from build123d import *

# Parameters (mm, degrees)
SKETCH1_R           = 2.5
SKETCH1_R_2         = 1.5
BOSS_EXTRUDE1_DEPTH = 310
SKETCH2_R           = 1.503835311
BOSS_EXTRUDE2_DEPTH = 5
LPATTERN1_COUNT     = 3
LPATTERN1_PITCH     = 30
SKETCH3_R           = 1.791065429
BOSS_EXTRUDE3_DEPTH = 5


with BuildPart() as part:
    # Sketch1 → Boss-Extrude1 (new body)
    with BuildSketch(Plane(origin=(0, 0, 0), x_dir=(1, 0, 0), z_dir=(0, 1, 0))):
        Circle(SKETCH1_R)
        Circle(SKETCH1_R_2, mode=Mode.SUBTRACT)
    extrude(amount=BOSS_EXTRUDE1_DEPTH)

    # Sketch2 → Boss-Extrude2 (add)
    with BuildSketch(Plane.XY):
        with Locations((0, 84.914129816)):
            Circle(SKETCH2_R)
    boss_extrude2 = extrude(amount=BOSS_EXTRUDE2_DEPTH)

    # LPattern1: Boss-Extrude2 ×3
    with Locations(*[(0, i * LPATTERN1_PITCH, 0) for i in range(1, LPATTERN1_COUNT)]):
        add(boss_extrude2)

    # Sketch3 → Boss-Extrude3 (add)
    with BuildSketch(Plane.XY):
        with Locations((0, 273.450822339)):
            Circle(SKETCH3_R)
    extrude(amount=BOSS_EXTRUDE3_DEPTH)


solid = part.part
CAD build for the part. Positions are in the model's coordinates, mm. A direction names the side the tool comes from. Coordinates: 2 decimals unless noted, no trailing zeros. Write each loop counter-clockwise with the first axis right and the second up, starting at its lowest first coordinate (ties: lowest second). Pieces come first, ordered by that corner, then holes. Notation, with made-up numbers: M 24,67 L 74,67 A9 cw 74,77 Z; hole C 88,7.25 d7. An arc over 180 degrees is marked long. Answer as a JSON object with one key per item and string values. Group by question number.
1) Pin check, flat tips, straight feed: pin 1 Ø2.5 at (x, z) = (0, 0) entering from -Y; pin 2 Ø3 at (x, y) = (1, 48.5) entering from +Z; pin 3 Ø1 at (x, y) = (-1, 249.5) entering from +Z. Stop position of each tip, or through.
2) Tool access for faces 1 (the face through (1.34, 152.83, -2.11)), 2 (the face through (0, 310, 2)): list every direction of +Z, -Z, +X, -X, +Y, -Y with a clear straight run to the whole face (end or side of a thin tool).
3) Wall check: line 1 (Z direction, x = 0.4, y = 29); line 2 (Z direction, x = 0, y = 179); line 3 (Y direction, x = 0.35, z = 4.75). Give the ranges that are in metal, low to high. Write a range as from..to.
4) Saw through at A-A (y = 31). Write the cut outline in (x, z).
Values follow:
{
 "1": {"pin 1": "stops at y = 83.41", "pin 2": "stops at z = 2.5", "pin 3": "stops at z = 2.45"},
 "2": {"face 1": "none", "face 2": "+Z, -Z, +X, -X, +Y"},
 "3": {"line 1": "z = -2.47..-1.45, 1.45..2.47", "line 2": "z = -2.5..-1.5, 1.5..2.5", "line 3": "y = 83.45..86.38, 113.45..116.38, 143.45..146.38, 271.69..275.21"},
 "4": {"outline": "C 0,0 d5; hole C 0,0 d3"}
}
